Verification items for the finished model (mm, model axes). A direction names the side the tool comes from. Give positions to 0.01 mm unless a question says otherwise; leave off trailing zeros. Write each loop counter-clockwise with the first axis right and the second up, starting at its lowest first coordinate (ties: lowest second). Pieces come first, ordered by that corner, then holes.
from build123d import *

# Parameters (mm, degrees)
PAD003_DEPTH    = 1.44
POCKET004_DEPTH = 9.75
POCKET005_DEPTH = 8.570714
CHAMFER002_SIZE = 0.5


with BuildPart() as part:
    # Sketch010 → Pad003 (new body)
    with BuildSketch(Plane.XZ):
        Polygon((-4.284857, 0), (4.284857, 0), (4.284857, 9.75), (4.284857, 39), (-4.284857, 39), (-4.284857, 9.75), align=None)
    extrude(amount=PAD003_DEPTH)

    # Sketch011 (on Face1 of Pad003) → Pocket004 (cut)
    with BuildSketch(Plane(origin=(0, 0, 0), x_dir=(1, 0, 0), z_dir=(0, 0, -1))):
        Polygon((-3.284857, 1.44), (-3.284857, 1), (-8.284857, 1), (-8.284857, 4.941038), align=None)
        Polygon((8.284857, 4.941038), (3.284857, 1.44), (3.284857, 1), (8.284857, 1), align=None)
    extrude(amount=-POCKET004_DEPTH, mode=Mode.SUBTRACT)

    # Sketch012 (on Face9 of Pocket004) → Pocket005 (cut, through all)
    with BuildSketch(Plane(origin=(-4.284857, 0, 0), x_dir=(0, 0, -1), z_dir=(-1, 0, 0))):
        Polygon((-39.051991, 0.21), (-10.038814, 1.44), (-39.051991, 14.04), align=None)
    extrude(amount=-POCKET005_DEPTH, mode=Mode.SUBTRACT)

    # Chamfer002
    chamfer002_edges = [part.edges().sort_by_distance(p)[0] for p in [
        (-3.784857, -1, 0),
        (-3.284857, -1.22, 0),
        (0, -1.44, 0),
        (3.284857, -1.22, 0),
        (3.784857, -1, 0),
        (-4.284857, -0.5, 0),
        (4.284857, -0.5, 0),
    ]]
    chamfer(chamfer002_edges, length=CHAMFER002_SIZE)


with BuildPart() as part_1:
    # Body001 placement: moved
    add(part.part.moved(Location((0, 25, 0))))


solid = part_1.part
Item 1: Set-up check for faces 1 (the face through (-4, 24, 5)), 2 (the face through (4, 24, 5)), 3 (the face through (-0.06, 24.182, 24.722)): record each of +Z, -Z, +X, -X, +Y, -Y from which the full face is reachable in a straight line by a thin tool's end or side.
Answer key:
face 1: -Z, -X, -Y
face 2: -Z, +X, -Y
face 3: +Z, +X, -X, -Y
Item 2: Scan lines: line 1 along Y through (x, z) = (3.75, 8.5); line 2 along Y through (x, z) = (4, 17). Record each from-to range of solid material in increasing order.
Answer key:
line 1: y = 24 to 25
line 2: y = 23.86 to 25
Item 3: Sectioned sample at D-D on z = 19. Record the cut outline in (x, y), then the cut area to 3 significant figures.
Answer key:
outline: (-4.28, 23.94) - (4.28, 23.94) - (4.28, 25) - (-4.28, 25) - close
area: 9.08 mm2
Item 4: Sectioned sample at B-B on x = 1.5. Record the cut outline in (y, z).
Answer key:
outline: (23.56, 0.5) - (24.06, 0) - (25, 0) - (25, 39) - (24.79, 39) - (23.56, 10.04) - close
Item 5: Sectioned sample at A-A on z = 6. Record the cut outline in (x, y), then the cut area to 3 significant figures.
Answer key:
outline: (-4.28, 24) - (-3.28, 24) - (-3.28, 23.56) - (3.28, 23.56) - (3.28, 24) - (4.28, 24) - (4.28, 25) - (-4.28, 25) - close
area: 11.5 mm2
Item 6: Sectioned sample at C-C on z = 36. Record the cut outline in (x, y).
Answer key:
outline: (-4.28, 24.66) - (4.28, 24.66) - (4.28, 25) - (-4.28, 25) - close
Item 7: Depth check by flat-ended pin: pin 1 (0.5 mm diameter, centred on x = -3.5, y = 24, fed in from -Z). Enter the tip coordinate at first touch or a pass-through.
Answer key:
pin 1: stops at z = 0.25
